```python
from build123d import *

# Parameters (mm, degrees)
F0_R     = 11.2
F1_DEPTH = 7


with BuildPart() as f1:
    # F0 (on Top) → F1 (new body)
    with BuildSketch(Plane.XY):
        with BuildLine():
            Line((19.215132, 22.378807), (0, 55.077419))
            Line((0, 55.077419), (-19.066227, 22.201317))
            ThreePointArc((-19.066227, 22.201317), (-15.219751, 8.713844), (-28.836632, 5.354102))
            Line((-28.836632, 5.354102), (-48.016034, -27.717147))
            Line((-48.016034, -27.717147), (-9.689672, -27.717147))
            ThreePointArc((-9.689672, -27.717147), (0.044547, -17.537595), (9.778766, -27.717147))
            Line((9.778766, -27.717147), (48.653703, -27.717147))
            Line((48.653703, -27.717147), (29.068287, 5.61158))
            ThreePointArc((29.068287, 5.61158), (15.203422, 8.742665), (19.215132, 22.378807))
        make_face()
        with Locations((-24.390228, -14.081704)):
            Circle(F0_R, mode=Mode.SUBTRACT)
        Circle(F0_R, mode=Mode.SUBTRACT)
        with Locations((24.390229, -14.081704)):
            Circle(F0_R, mode=Mode.SUBTRACT)
        with Locations((0, 28.163411)):
            Circle(F0_R, mode=Mode.SUBTRACT)
    extrude(amount=F1_DEPTH)


solid = f1.part
```
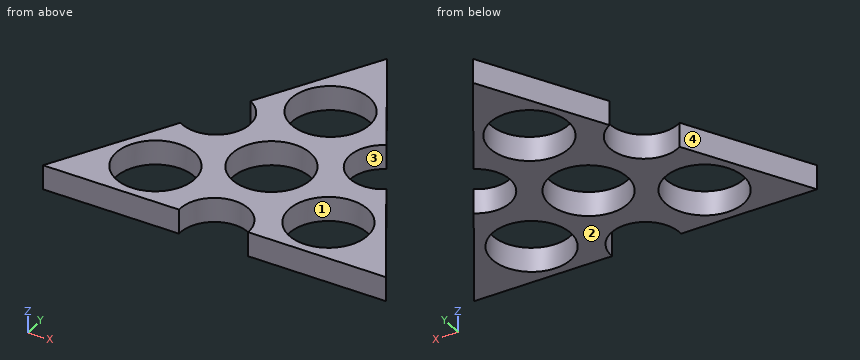
Design review of the part built by this model. Coordinates are the model's own, in mm. Face numbers are marked on the shaded views. Give positions to 0.01 mm unless a question says otherwise; leave off trailing zeros. Write each loop counter-clockwise with the first axis right and the second up, starting at its lowest first coordinate (ties: lowest second). Pieces come first, ordered by that corner, then holes. Notation, with made-up numbers: (-3, -35) - (32, -35) arc R30 cw to (32, -10) - close; hole circle Ø10 at (17.5, 65). An arc over 180 degrees is marked (long way). Return JSON: item names as keys, results as strings. Group by question number.
(1) Mouldability with a two-part tool opening along Y and no side actions: class the marked faces 1, 2, 3 and 4 as +Y half, -Y half, draft (parallel to the pull), parting line (faces both ways), or undercut.
(2) We need section B-B, the plane y = 0. Give the boundary of the cut face in (x, z), then the cut area to 3 significant figures.
(3) We need section D-D, the plane z = 3. Give the boundary of the cut face in (x, y), then the cut area to 3 significant figures.
(4) To check wall thickness, follow probe 1 along Y at (x, z) = (-3.5, 3.5); probe 2 along X at (y, z) = (-20, 2); probe 3 along Y at (x, z) = (-16, 2.5). State the ranges of each line that lie inside material, in increasing order.
(5) We need section C-C, the plane y = -21. Give the boundary of the cut face in (x, z).
(6) We need section A-A, the plane x = 18. Give the boundary of the cut face in (y, z).
Reported:
{
 "1": {"face 1": "undercut", "face 2": "draft", "face 3": "undercut", "face 4": "+Y half"},
 "2": {"outline": "(-31.94, 0) - (-11.2, 0) - (-11.2, 7) - (-31.94, 7) - close; (11.2, 0) - (32.37, 0) - (32.37, 7) - (11.2, 7) - close", "area": "293 mm2"},
 "3": {"outline": "(-48.02, -27.72) - (-9.69, -27.72) arc R9.74 cw (long way) to (9.78, -27.72) - (48.65, -27.72) - (29.07, 5.61) arc R9.74 cw (long way) to (19.22, 22.38) - (0, 55.08) - (-19.07, 22.2) arc R9.74 cw (long way) to (-28.84, 5.35) - close; hole circle Ø22.4 at (-24.39, -14.08); hole circle Ø22.4 at (0, 0); hole circle Ø22.4 at (0, 28.16); hole circle Ø22.4 at (24.39, -14.08)", "area": "1,950 mm2"},
 "4": {"probe 1": "y = -18.21 to -10.64, 10.64 to 17.52, 38.8 to 49.04", "probe 2": "x = -43.54 to -33.9, -14.88 to -6.43, 6.52 to 14.88, 33.9 to 44.12", "probe 3": "y = -27.72 to -21.5, -6.66 to 7.57, 19.64 to 27.49"},
 "5": {"outline": "(-44.12, 0) - (-33.2, 0) - (-33.2, 7) - (-44.12, 7) - close; (-15.58, 0) - (-7.4, 0) - (-7.4, 7) - (-15.58, 7) - close; (7.49, 0) - (15.58, 0) - (15.58, 7) - (7.49, 7) - close; (33.2, 0) - (44.71, 0) - (44.71, 7) - (33.2, 7) - close"},
 "6": {"outline": "(-27.72, 0) - (-23.28, 0) - (-23.28, 7) - (-27.72, 7) - close; (-4.88, 0) - (5.71, 0) - (5.71, 7) - (-4.88, 7) - close; (21.65, 0) - (24.45, 0) - (24.45, 7) - (21.65, 7) - close"}
}
